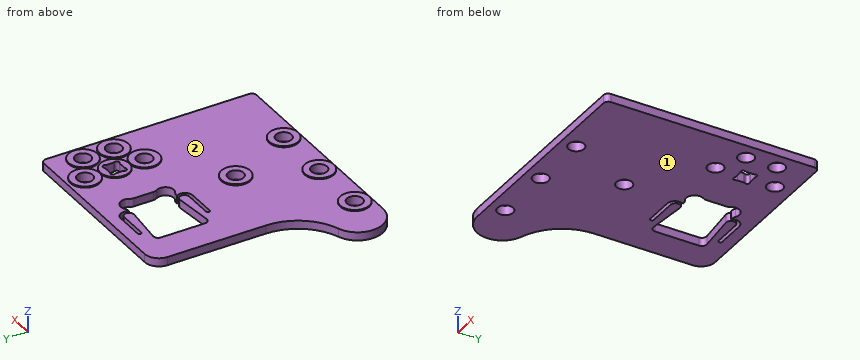
from build123d import *

# Parameters (mm, degrees)
SKETCH_R     = 6.6
PAD_DEPTH    = 8
SKETCH001_R  = 12.199475
POCKET_DEPTH = 1


with BuildPart() as part:
    # Sketch → Pad (new body)
    with BuildSketch(Plane.XY):
        with BuildLine():
            Line((-4, 40), (-146, 40))
            ThreePointArc((-146, 40), (-154.485281, 36.485281), (-158, 28))
            Line((-158, -55), (-158, 28))
            ThreePointArc((-188.565904, -97.622258), (-166.431336, -81.224661), (-158, -55))
            ThreePointArc((-188.565904, -97.622258), (-202.717412, -121.203739), (-181.74971, -139))
            Line((-181.74971, -139), (-4, -139))
            ThreePointArc((-4, -139), (-1.171573, -137.828427), (0, -135))
            Line((0, 36), (0, -135))
            ThreePointArc((0, 36), (-1.171573, 38.828427), (-4, 40))
        make_face()
        with Locations((-37, 25)):
            Circle(SKETCH_R, mode=Mode.SUBTRACT)
        with Locations((-37, -25)):
            Circle(SKETCH_R, mode=Mode.SUBTRACT)
        with Locations((-14, 13)):
            Circle(SKETCH_R, mode=Mode.SUBTRACT)
        with Locations((-14, -13)):
            Circle(SKETCH_R, mode=Mode.SUBTRACT)
        with Locations((-164, -126)):
            Circle(SKETCH_R, mode=Mode.SUBTRACT)
        with Locations((-114, -126)):
            Circle(SKETCH_R, mode=Mode.SUBTRACT)
        with Locations((-64, -126)):
            Circle(SKETCH_R, mode=Mode.SUBTRACT)
        with Locations((-90.2, -70)):
            Circle(SKETCH_R, mode=Mode.SUBTRACT)
        with BuildLine():
            Line((-40.101765, 6.2), (-33.898235, 6.2))
            ThreePointArc((-33.898235, 6.2), (-33.357039, 6.274615), (-32.856224, 6.492893))
            ThreePointArc((-30.107107, 3.743776), (-30.4, 6.2), (-32.856224, 6.492893))
            ThreePointArc((-30.107107, 3.743776), (-30.325385, 3.242961), (-30.4, 2.701765))
            Line((-30.4, 2.701765), (-30.4, -2.701765))
            ThreePointArc((-30.4, -2.701765), (-30.325385, -3.242961), (-30.107107, -3.743776))
            ThreePointArc((-32.856224, -6.492893), (-30.4, -6.2), (-30.107107, -3.743776))
            ThreePointArc((-32.856224, -6.492893), (-33.357039, -6.274615), (-33.898235, -6.2))
            Line((-33.898235, -6.2), (-40.101765, -6.2))
            ThreePointArc((-40.101765, -6.2), (-40.642961, -6.274615), (-41.143776, -6.492893))
            ThreePointArc((-43.892893, -3.743776), (-43.6, -6.2), (-41.143776, -6.492893))
            ThreePointArc((-43.892893, -3.743776), (-43.674615, -3.242961), (-43.6, -2.701765))
            Line((-43.6, -2.701765), (-43.6, 2.701765))
            ThreePointArc((-43.6, 2.701765), (-43.674615, 3.242961), (-43.892893, 3.743776))
            ThreePointArc((-41.143776, 6.492893), (-43.6, 6.2), (-43.892893, 3.743776))
            ThreePointArc((-41.143776, 6.492893), (-40.642961, 6.274615), (-40.101765, 6.2))
        make_face(mode=Mode.SUBTRACT)
        with BuildLine():
            Line((-90.7, 20.3), (-89.943823, 20.3))
            ThreePointArc((-89.943823, 20.3), (-88.049637, 20.561153), (-86.296785, 21.325126))
            ThreePointArc((-76.674874, 11.703215), (-77.700001, 20.3), (-86.296785, 21.325126))
            ThreePointArc((-76.674874, 11.703215), (-77.438847, 9.950364), (-77.7, 8.056178))
            Line((-77.7, 8.056178), (-77.7, -8.056178))
            ThreePointArc((-77.7, -8.056178), (-77.438847, -9.950365), (-76.674874, -11.703216))
            ThreePointArc((-86.296785, -21.325126), (-77.7, -20.3), (-76.674874, -11.703216))
            ThreePointArc((-86.296785, -21.325126), (-88.049636, -20.561153), (-89.943822, -20.3))
            Line((-90.7, -20.3), (-89.943822, -20.3))
            ThreePointArc((-96.2, -30.280093), (-90.502363, -26.91448), (-90.7, -20.3))
            Line((-96.2, -30.280093), (-120, -30.280093))
            ThreePointArc((-120, -27.280093), (-121.5, -28.780093), (-120, -30.280093))
            Line((-96.2, -27.280093), (-120, -27.280093))
            ThreePointArc((-96.2, -27.280093), (-92.20498, -23.080559), (-96.598572, -19.3))
            Line((-128.601428, -22.504808), (-96.598572, -19.3))
            ThreePointArc((-133, -18.524715), (-131.683814, -21.490713), (-128.601428, -22.504808))
            Line((-133, 18.524715), (-133, -18.524715))
            ThreePointArc((-128.601428, 22.504808), (-131.683814, 21.490713), (-133, 18.524715))
            Line((-128.601428, 22.504808), (-96.598572, 19.3))
            ThreePointArc((-96.598572, 19.3), (-92.20498, 23.080559), (-96.2, 27.280093))
            Line((-96.2, 27.280093), (-120, 27.280093))
            ThreePointArc((-120, 30.280093), (-121.5, 28.780093), (-120, 27.280093))
            Line((-96.2, 30.280093), (-120, 30.280093))
            ThreePointArc((-90.7, 20.3), (-90.502363, 26.91448), (-96.2, 30.280093))
        make_face(mode=Mode.SUBTRACT)
    extrude(amount=-PAD_DEPTH)

    # Sketch001 → Pocket (cut)
    with BuildSketch(Plane.XY):
        Polygon((5.517247, 44.094818), (5.517247, -142.525909), (-211.650055, -142.525909), (-211.650055, -44.465102), (-211.650055, 44.094818), align=None)
        with Locations((-37, -25)):
            Circle(SKETCH001_R, mode=Mode.SUBTRACT)
        with Locations((-14, 13)):
            Circle(SKETCH001_R, mode=Mode.SUBTRACT)
        with Locations((-14, -13)):
            Circle(SKETCH001_R, mode=Mode.SUBTRACT)
        with Locations((-37, 25)):
            Circle(SKETCH001_R, mode=Mode.SUBTRACT)
        with Locations((-114, -126)):
            Circle(SKETCH001_R, mode=Mode.SUBTRACT)
        with Locations((-90.2, -70)):
            Circle(SKETCH001_R, mode=Mode.SUBTRACT)
        with Locations((-64, -126)):
            Circle(SKETCH001_R, mode=Mode.SUBTRACT)
        with Locations((-164, -126)):
            Circle(SKETCH001_R, mode=Mode.SUBTRACT)
        with Locations((-37, 0)):
            Circle(SKETCH001_R, mode=Mode.SUBTRACT)
    extrude(amount=-POCKET_DEPTH, mode=Mode.SUBTRACT)


solid = part.part
The listing builds one solid part. Answer for the finished solid, in the listing's coordinates (mm). Face numbers are marked on the shaded views. A direction names the side the tool comes from. Coordinates: 2 decimals unless noted, no trailing zeros. Order: outer loops, then holes, each group sorted by start corner. A loop starts at its lowest first (then second) coordinate and runs counter-clockwise, first axis right, second up.
Q1. A cutting plane is placed at C-C, the plane y = -73. Write down the section's boundary in (x, z), and give its area (3 significant figures).
Q2. Which of the six approach directions +Z, -Z, +X, -X, +Y, -Y give full straight-line access (tool end or side, diameter ignored) to the marked faces 1 and 2?
Q3. Given P1, Ø1.6, axis at y = 0, z = -3, coming from the -X side; P2, Ø4, axis at y = -85, z = -5.5, coming from the -X side; P3, Ø8, axis at x = -90.2, y = -70, coming from the +Z side, each flat-ended and moving along its own axis, determine where each tip first touches the part or whether it passes through.
Q4. A cutting plane is placed at A-A, the plane x = -64. Write down the section's boundary in (y, z).
Q5. Consider line 1 (Y direction, x = -37, z = -3); line 2 (X direction, y = -19, z = -5); line 3 (Y direction, x = -11, z = -2). Determine where each line is inside the solid, lowest interval first.
Q6. A cutting plane is placed at B-B, the plane y = -123.5. Write down the section's boundary in (x, z).
Q7. A cutting plane is placed at D-D, the plane z = -2.75. State how many separate pieces and enclosed holes the cut face has, and give its area (3 significant figures).
Answers follow:
1. outline: (-161.76, -8) - (-96.08, -8) - (-96.08, 0) - (-102.02, 0) - (-102.02, -1) - (-161.76, -1) - close; (-84.32, -8) - (0, -8) - (0, -1) - (-78.38, -1) - (-78.38, 0) - (-84.32, 0) - close
1. area: 1,060 mm2
2. face 1: -Z, +X, -X, +Y, -Y
2. face 2: +Z
3. P1: stops at x = -158
3. P2: stops at x = -171.36
3. P3: passes through
4. outline: (-139, -8) - (-132.6, -8) - (-132.6, 0) - (-138.2, 0) - (-138.2, -1) - (-139, -1) - close; (-119.4, -8) - (40, -8) - (40, -1) - (-113.8, -1) - (-113.8, 0) - (-119.4, 0) - close
5. line 1: y = -139 to -31.6, -18.4 to -6.2, 6.2 to 18.4, 31.6 to 40
5. line 2: x = -158 to -132.97, -76.68 to -39.75, -34.25 to -16.75, -11.25 to 0
5. line 3: y = -139 to -18.88, -7.12 to 7.12, 18.88 to 40
6. outline: (-202.21, -8) - (-170.11, -8) - (-170.11, 0) - (-175.94, 0) - (-175.94, -1) - (-202.21, -1) - close; (-157.89, -8) - (-120.11, -8) - (-120.11, 0) - (-125.94, 0) - (-125.94, -1) - (-152.06, -1) - (-152.06, 0) - (-157.89, 0) - close; (-107.89, -8) - (-70.11, -8) - (-70.11, 0) - (-75.94, 0) - (-75.94, -1) - (-102.06, -1) - (-102.06, 0) - (-107.89, 0) - close; (-57.89, -8) - (0, -8) - (0, -1) - (-52.06, -1) - (-52.06, 0) - (-57.89, 0) - close
7. separate pieces: 1
7. enclosed holes: 10
7. area: 26,500 mm2
